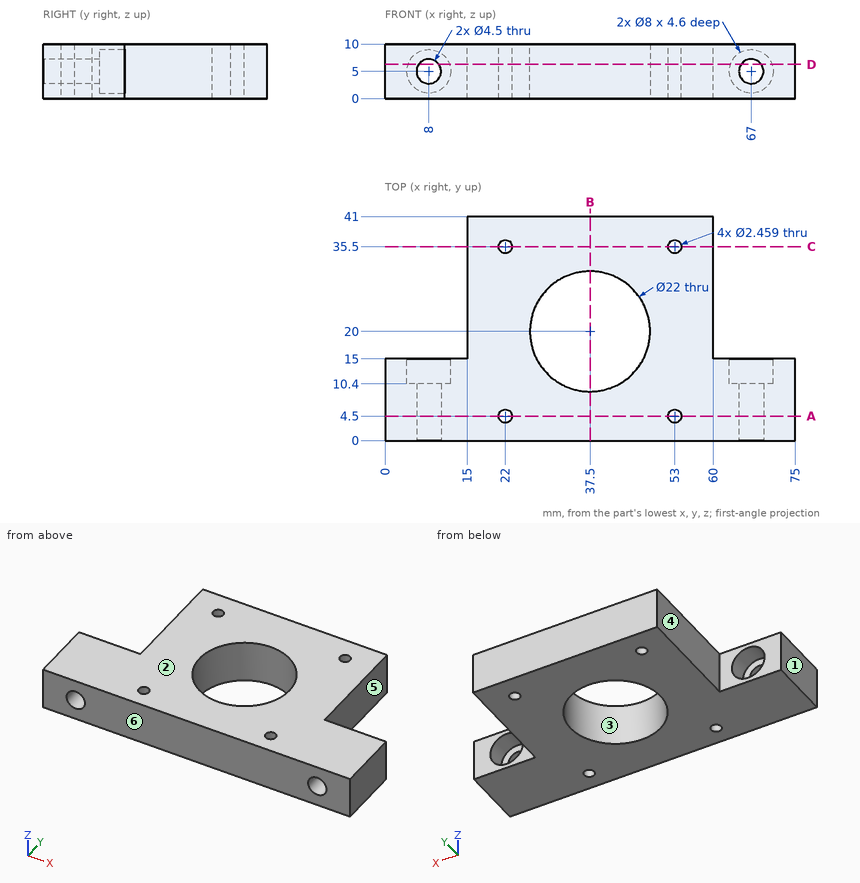
The drawing under review shows one solid part. Ordinate dimensions are in mm from its lowest x, y, z. A direction names the side the tool comes from. Give positions to 0.01 mm unless a question says otherwise; leave off trailing zeros. Loops run counter-clockwise (first coordinate to the right, second up) from the corner with the lowest first, then second, coordinate; pieces in that order, holes last. Notation, with made-up numbers: M 80.5,10.25 L 86.5,10.25 A27 cw 86.5,37.25 Z; hole C 71.25,-39.5 d1. An arc over 180 degrees is marked long. One line per item, written item: value. Start each with the question number.
Q1. Add section D-D (z = 6.25). Count the separate pieces of the cut face and the enclosed holes in it, and give its area (3 significant figures).
Q2. Machinability: for the marked faces 4, 5 and 6, which of the approach directions +Z, -Z, +X, -X, +Y, -Y give a long, thin tool a straight path to every point of the face, cutting with its end or side? Answer none if there is none.
Q3. Clearance check with a flat-ended pin moving along its axis: pin 1 Ø5 at (y, z) = (33, 3.5) entering from -X. State where the tip first meets the part, or that it passes through.
Q4. Add section C-C (y = 35.5). Give the boundary of the cut face in (x, z).
Q5. Draft analysis for pull direction X (two halves, no side actions). For the marked faces 1, 2 and 3, state which applies: released by +X, released by -X, zero draft, split by the parting line, or undercut.
Q6. Add section B-B (x = 37.5). Give the boundary of the cut face in (y, z).
Q7. Add section A-A (y = 4.5). Give the boundary of the cut face in (x, z).
Q8. For L1, parallel to Z at x = 8, y = 13.6; L2, parallel to X at y = 4, z = 1.5; L3, parallel to Y at x = 23, z = 2, list the stretches that pass through material, from the lowest coordinate up.
Reply:
1. separate pieces: 3
1. enclosed holes: 5
1. area: 1,750 mm²
2. face 4: +Z, -Z, -X, +Y
2. face 5: +Z, -Z, +X, +Y
2. face 6: +Z, -Z, +X, -X, -Y
3. pin 1: x = 15
4. outline: M 15,0 L 20.77,0 L 20.77,10 L 15,10 Z; M 23.23,0 L 51.77,0 L 51.77,10 L 23.23,10 Z; M 54.23,0 L 60,0 L 60,10 L 54.23,10 Z
5. face 1: released by -X
5. face 2: zero draft
5. face 3: undercut
6. outline: M 0,0 L 9,0 L 9,10 L 0,10 Z; M 31,0 L 41,0 L 41,10 L 31,10 Z
7. outline: M 0,0 L 20.77,0 L 20.77,10 L 0,10 Z; M 23.23,0 L 51.77,0 L 51.77,10 L 23.23,10 Z; M 54.23,0 L 75,0 L 75,10 L 54.23,10 Z; hole C 8,5 d4.5; hole C 67,5 d4.5
8. L1: 0 to 1, 9 to 10
8. L2: 0 to 20.88, 23.12 to 51.88, 54.12 to 75
8. L3: 0 to 3.78, 5.22 to 34.78, 36.22 to 41
